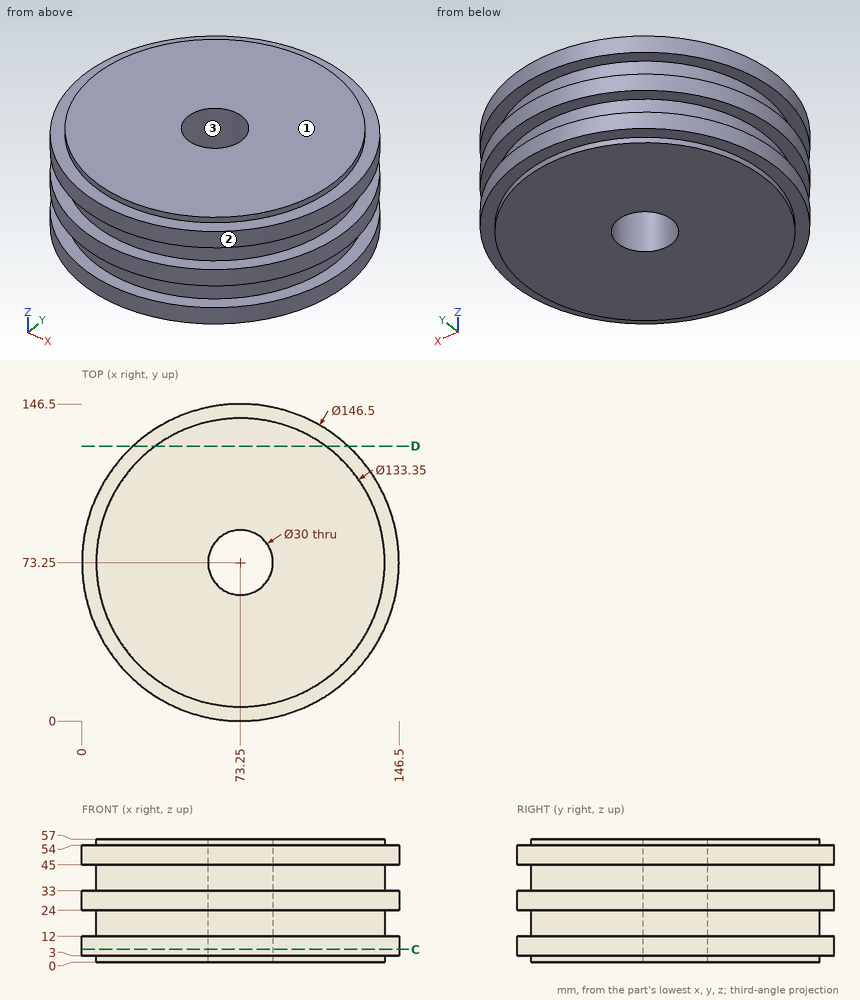
Study the drawing (mm; zero at the part's minimum x, y, z) and answer. Give positions to 0.01 mm unless a question says otherwise; leave off trailing zeros. Loops run counter-clockwise (first coordinate to the right, second up) from the corner with the lowest first, then second, coordinate; pieces in that order, holes last. Notation, with made-up numbers: (23, -25.75) - (56, -25.75) arc R33 cw to (56, 12.25) - close; hole circle Ø7 at (43, -8). An arc over 180 degrees is marked (long way). Answer in a Markdown table with one row per item. Add a question column.
Q1. The part is cut by section D-D (y = 127). Determine the outline of the cut face in (x, z), and give its area (3 significant figures).
Q2. Consider line 1 along Y through (x, z) = (73, 40); line 2 along Y through (x, z) = (73, 32); line 3 along X through (y, z) = (87, 21). Determine where each line is inside the solid, lowest interval first.
Q3. The part is cut by section C-C (z = 6). Determine the outline of the cut face in (x, y), and give its area (3 significant figures).
Q4. Determine the mould class of the marked faces 1, 2 and 3 for opening direction Y: released by +Y, released by -Y, zero draft, split by the parting line, or undercut.
Q5. Each of these flat-tipped pins is pushed along its axis until it touches: P1, Ø2, axis at y = 37, z = 36, coming from the +X side (3 decimals); P2, Ø1, axis at x = 48, z = 45.5, coming from the -Y side; P3, Ø8, axis at x = 113, z = 29.5, coming from the -Y side; P4, Ø6, axis at x = 116.5, y = 123.5, coming from the -Z side. Where does it stop, or does it pass through?
Solution:
| question | item | result |
|---|---|---|
| 1 | outline | (23.49, 3) - (33.8, 3) - (33.8, 0) - (112.7, 0) - (112.7, 3) - (123.01, 3) - (123.01, 12) - (112.7, 12) - (112.7, 24) - (123.01, 24) - (123.01, 33) - (112.7, 33) - (112.7, 45) - (123.01, 45) - (123.01, 54) - (112.7, 54) - (112.7, 57) - (33.8, 57) - (33.8, 54) - (23.49, 54) - (23.49, 45) - (33.8, 45) - (33.8, 33) - (23.49, 33) - (23.49, 24) - (33.8, 24) - (33.8, 12) - (23.49, 12) - close |
| 1 | area | 5,050 mm² |
| 2 | line 1 | y = 6.58 to 58.25, 88.25 to 139.92 |
| 2 | line 2 | y = 0 to 58.25, 88.25 to 146.5 |
| 2 | line 3 | x = 8.01 to 67.26, 79.24 to 138.49 |
| 3 | outline | circle Ø146.5 at (73.25, 73.25); hole circle Ø30 at (73.25, 73.25) |
| 3 | area | 16,100 mm² |
| 4 | face 1 | zero draft |
| 4 | face 2 | split by the parting line |
| 4 | face 3 | undercut |
| 5 | P1 | stops at x = 129.845 |
| 5 | P2 | stops at y = 4.31 |
| 5 | P3 | stops at y = 9.32 |
| 5 | P4 | stops at z = 0 |
